Check sheet for the modelled part. Datum: model origin and axes. Units: mm. A direction names the side the tool comes from. Coordinates: 2 decimals unless noted, no trailing zeros. Loops run counter-clockwise (first coordinate to the right, second up) from the corner with the lowest first, then second, coordinate; pieces in that order, holes last. Notation, with made-up numbers: (80, -4) - (113, -4) arc R21 cw to (113, 2) - close; hole circle Ø8 at (-20, -16.5). An arc over 180 degrees is marked (long way). Use a Markdown table: item, result. Add a question column.
1) Go/stop test with flat-tipped pins: P1, Ø4, axis at x = -53, y = -3, coming from the +Z side; P2, Ø6, axis at x = -15, y = -13, coming from the -Z side; P3, Ø5, axis at x = -67, z = 19.5, coming from the +Y side; P4, Ø13.5, axis at y = -19, z = 25, coming from the +X side. Record where each tip stops, or that it passes through.
2) Draft check along X on faces 6 (the flat face through (-43, -14, -5)), 7 (the flat face through (-10, -15, 4)), 8 (the flat face through (0, 25, 0)). Enter one of: pulls with the +X half, pulls with the -X half, needs draft (parallel to the pull), parting line crosses it, or undercut.
3) Tool access check on faces 1 (the flat face through (-16, -18, 8)), 2 (the cylindrical face through (-68, -19, 36)), 3 (the cylindrical face through (8.716, -28.706, -0.112)), 4 (the cylindrical face through (-15.035, -16.061, 5.479)), 5 (the cylindrical face through (-15.035, -16.061, -5.521)). Record the directions out of +Z, -Z, +X, -X, +Y, -Y that give a thin tool (end or side, any length) a straight path to the whole face; none if there is none.
4) Sectioned sample at C-C, the plane z = 11. Enter the section's corners in (x, y), then the cut area to 3 significant figures.
5) Sectioned sample at B-B, the plane x = -41. Enter the section's corners in (y, z), then the cut area to 3 significant figures.
6) Sectioned sample at A-A, the plane z = -1.5. Enter the section's corners in (x, y), then the cut area to 3 significant figures.
7) Thickness scan on line 1 (Z direction, x = -69, y = -19); line 2 (Y direction, x = -66.25, z = 25); line 3 (Z direction, x = -32, y = -23). Record the ranges inside material, lowest first.
Autodesk Inventor part; units mm, degrees
ref_plane "YZ Plane" through (0, 0, 0) normal (1, 0, 0) x (0, 1, 0)
ref_plane "XZ Plane" through (0, 0, 0) normal (0, 1, 0) x (-1, 0, 0)
ref_plane "XY Plane" through (0, 0, 0) normal (0, 0, 1) x (1, 0, 0)
sketch "스케치1" plane through (0, 0, 0) normal (0, 1, 0) x (-1, 0, 0)
  point P0 (0, 0)
sketch "스케치2" plane through (0, 0, 0) normal (0, 0, 1) x (1, 0, 0)
  arc A0 (0, 16) -> (16, 0) centre (0, 0) ccw
  arc A1 (0, 22) -> (22, 0) centre (0, 0) ccw
  arc A2 (0, 30) -> (30, 0) centre (0, 0) ccw
  line L0 (-70, -8) -> (-60, -8)
  line L1 (-60, -8) -> (-60, -30)
  line L2 (-60, -30) -> (-70, -30)
  line L3 (-70, -30) -> (-70, -8)
  line L4 (-70, -8) -> (-15.7735, 25.5185)
  line L5 (-70, -30) -> (0, -30)
  line L6 (-73, -8) -> (-70, -8)
  line L7 (-73, -8) -> (-73, -30)
  line L8 (-67, -30) -> (-73, -30)
  line L9 (0, 40) -> (0, -40)
  line L10 (-40, 0) -> (40, 0)
  point P0 (-71.5, -8)
  dimension "d0" = 32
  dimension "d1" = 44
  dimension "d2" = 60
  dimension "d4" = 22
  dimension "d5" = 70
  dimension "d7" = 10
  dimension "d8" = 3
  dimension "d13" = 80
  dimension "d14" = 80
extrude "돌출3" add sketch "스케치2" along normal mid plane 8 contours A0 L10 A1 L9 | A0 L9 A1 L10 | A0 L10 A1 L9
extrude "돌출4" add sketch "스케치2" along normal mid plane 16 contours A1 L10 A2 L9 | A1 L9 A2 L10 | A1 L10 A2 L9
extrude "돌출5" add sketch "스케치2" along normal mid plane 10 contours A2 L5 L1 L0 L4
extrude "돌출6" add sketch "스케치2" against normal blind 5 contours L0 L1 L2 L3
extrude "돌출7" add sketch "스케치2" along normal blind 25 contours L0 L1 L2 L3
sketch "스케치4" plane through (-60, -30, 5) normal (1, 0, 0) x (0, 0, -1)
  circle A0 centre (-20, 11) radius 11
  circle A1 centre (-20, 11) radius 7.5
  line L0 (-20, 0) -> (-20, 22)
  line L1 (10, 0) -> (10, 55.5185)
  line L2 (10, 0) -> (-20, 0)
  line L3 (10, 22) -> (-20, 22)
  point P0 (5, 30)
  point P1 (-5, 0)
  point P2 (-20, 18.5)
  point P3 (-20, 3.5)
  dimension "d28" = 22
  dimension "d29" = 15
  dimension "d30" = 30
extrude "돌출8" add sketch "스케치4" against normal blind 13 contours A0 L0 A1 | L0 A1 A0
extrude "돌출9" cut sketch "스케치4" against normal blind 13 contours A1 L0 picked at (-15.876, 12.5587)
fillet "모깎기1" radius 1 6 edges at (-11.3137, -11.3137, 4) (-15.5563, -15.5563, 8) (-60, -11.5, 25) (-11.3137, -11.3137, -4) (-15.5563, -15.5563, -8) (-73, -19, 32.5)
properties part number "Day02_Task02"
Solved:
| question | item | result |
|---|---|---|
| 1 | P1 | stops at z = 5 |
| 1 | P2 | stops at z = -7.99 |
| 1 | P3 | stops at y = -8 |
| 1 | P4 | passes through |
| 2 | face 6 | needs draft |
| 2 | face 7 | undercut |
| 2 | face 8 | pulls with the +X half |
| 3 | face 1 | +Z, +X, +Y, -Y |
| 3 | face 2 | -X |
| 3 | face 3 | none |
| 3 | face 4 | +Z |
| 3 | face 5 | -Z |
| 4 | outline | (-70, -30) - (-60, -30) - (-60, -8) - (-70, -8) - close |
| 4 | area | 220 mm2 |
| 5 | outline | (-30, -5) - (9.93, -5) - (9.93, 5) - (-30, 5) - close |
| 5 | area | 399 mm2 |
| 6 | outline | (-70, -30) - (0, -30) arc R30 ccw to (30, 0) - (16, 0) arc R16 cw (long way) to (0, 16) - (0, 30) arc R30 ccw to (-15.77, 25.52) - (-70, -8) - close |
| 6 | area | 3,130 mm2 |
| 7 | line 1 | z = -5 to 17.5, 32.5 to 36 |
| 7 | line 2 | y = -30 to -26.5, -11.5 to -8 |
| 7 | line 3 | z = -5 to 5 |
